Verification items for the finished model (mm, model axes). Coordinates: 2 decimals unless noted, no trailing zeros. Order: outer loops, then holes, each group sorted by start corner. A loop starts at its lowest first (then second) coordinate and runs counter-clockwise, first axis right, second up. Notation, with made-up numbers: M 27.5,36 L 69.5,36 A17 ccw 69.5,64 Z; hole C -17.75,-38.75 d10. An arc over 180 degrees is marked long. Return JSON: item names as keys, results as strings.
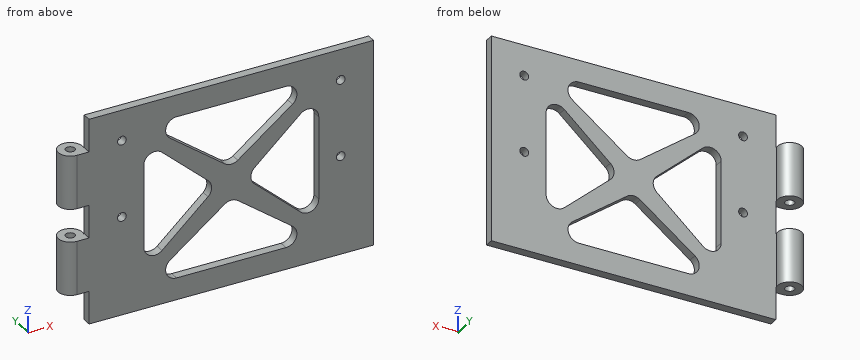
```python
from build123d import *

# Parameters (mm, degrees)
SKETCH_1_W           = 130
SKETCH_1_H           = 94
EXTRUDE_1_DEPTH      = 4
EXTRUDE_2_DEPTH      = 32
EXTRUDE_2_DEPTH_BACK = 32
SKETCH_4_R           = 2.1
CUT_EXTRUDE_1_DEPTH  = 122.379569945
SKETCH_10_W          = 11
SKETCH_10_H          = 15
CUT_EXTRUDE_2_DEPTH  = 24
CUT_EXTRUDE_3_DEPTH  = 10
SKETCH_12_R          = 2
CUT_EXTRUDE_4_DEPTH  = 10


with BuildPart() as part:
    # Эскиз1 → Бобышка-Вытянуть1 (new body)
    with BuildSketch(Plane(origin=(0, 0, 0), x_dir=(1, 0, 0), z_dir=(0, 1, 0))):
        Rectangle(SKETCH_1_W, SKETCH_1_H)
    extrude(amount=EXTRUDE_1_DEPTH)

    # Эскиз2 → Бобышка-Вытянуть2 (add, two sides: drawn at the far end of the back side and taken through both)
    with BuildSketch(Plane.XY.offset(-EXTRUDE_2_DEPTH_BACK)):
        with BuildLine():
            Line((-65, 4), (-65.208497378, 4))
            ThreePointArc((-65.208497378, 4), (-73.81662479, 9.887482194), (-70.5, 0))
            Line((-70.5, 0), (-65, 0))
            Line((-65, 0), (-65, 4))
        make_face()
    extrude(amount=EXTRUDE_2_DEPTH + EXTRUDE_2_DEPTH_BACK)

    # Эскиз4 → Вырез-Вытянуть1 (cut, through all)
    with BuildSketch(Plane.XY.offset(47)):
        with Locations((-70.5, 5.5)):
            Circle(SKETCH_4_R)
    extrude(amount=-CUT_EXTRUDE_1_DEPTH, mode=Mode.SUBTRACT)

    # Эскиз10 → Вырез-Вытянуть2 (cut)
    with BuildSketch(Plane(origin=(0, 0, 0), x_dir=(1, 0, 0), z_dir=(0, 1, 0))):
        with Locations((-70.5, 0)):
            Rectangle(SKETCH_10_W, SKETCH_10_H)
    extrude(amount=CUT_EXTRUDE_2_DEPTH, mode=Mode.SUBTRACT)

    # Эскиз11 → Вырез-Вытянуть3 (cut)
    with BuildSketch(Plane(origin=(0, 4, 0), x_dir=(1, 0, 0), z_dir=(0, 1, 0))):
        with BuildLine():
            Line((-25, 37), (25, 37))
            ThreePointArc((25, 37), (29.74341649, 33.58113883), (28, 28))
            Line((28, 28), (3, 9.25))
            ThreePointArc((3, 9.25), (0, 8.25), (-3, 9.25))
            Line((-3, 9.25), (-28, 28))
            ThreePointArc((-28, 28), (-29.74341649, 33.58113883), (-25, 37))
        make_face()
        with BuildLine():
            Line((-3, -9.25), (-28, -28))
            ThreePointArc((-28, -28), (-29.74341649, -33.58113883), (-25, -37))
            Line((-25, -37), (25, -37))
            ThreePointArc((25, -37), (29.74341649, -33.58113883), (28, -28))
            Line((28, -28), (3, -9.25))
            ThreePointArc((3, -9.25), (0, -8.25), (-3, -9.25))
        make_face()
        with BuildLine():
            Line((-10.625647004, 3.726779962), (-31.666666667, 22.546440075))
            ThreePointArc((-31.666666667, 22.546440075), (-37.041241452, 23.384014758), (-40, 18.819660113))
            Line((-40, 18.819660113), (-40, -18.819660113))
            ThreePointArc((-40, -18.819660113), (-37.041241452, -23.384014758), (-31.666666667, -22.546440075))
            Line((-31.666666667, -22.546440075), (-10.625647004, -3.726779962))
            ThreePointArc((-10.625647004, -3.726779962), (-8.958980338, 0), (-10.625647004, 3.726779962))
        make_face()
        with BuildLine():
            Line((10.625647004, 3.726779962), (31.666666667, 22.546440075))
            ThreePointArc((31.666666667, 22.546440075), (37.041241452, 23.384014758), (40, 18.819660113))
            Line((40, 18.819660113), (40, -18.819660113))
            ThreePointArc((40, -18.819660113), (37.041241452, -23.384014758), (31.666666667, -22.546440075))
            Line((31.666666667, -22.546440075), (10.625647004, -3.726779962))
            ThreePointArc((10.625647004, -3.726779962), (8.958980338, 0), (10.625647004, 3.726779962))
        make_face()
    extrude(amount=-CUT_EXTRUDE_3_DEPTH, mode=Mode.SUBTRACT)

    # Эскиз12 → Вырез-Вытянуть4 (cut)
    with BuildSketch(Plane(origin=(0, 4, 0), x_dir=(1, 0, 0), z_dir=(0, 1, 0))):
        with Locations(Location((-50, 2, 0), (0, 0, 270))):
            Circle(SKETCH_12_R)
        with Locations(Location((50, 2, 0), (0, 0, 270))):
            Circle(SKETCH_12_R)
        with Locations(Location((50, -33, 0), (0, 0, 270))):
            Circle(SKETCH_12_R)
        with Locations(Location((-50, -33, 0), (0, 0, 270))):
            Circle(SKETCH_12_R)
    extrude(amount=-CUT_EXTRUDE_4_DEPTH, mode=Mode.SUBTRACT)


solid = part.part
```
Q1. Cross-section at B-B, the plane y = 5.5. Record the boundary of the cut face in (x, z).
Values:
{"outline": "M -76,-32 L -72.6,-32 L -72.6,-7.5 L -76,-7.5 Z; M -76,7.5 L -72.6,7.5 L -72.6,32 L -76,32 Z; M -68.4,-32 L -65,-32 L -65,-7.5 L -68.4,-7.5 Z; M -68.4,7.5 L -65,7.5 L -65,32 L -68.4,32 Z"}
Q2. Cross-section at C-C, the plane z = -34. Record the boundary of the cut face in (x, y).
Values:
{"outline": "M -65,0 L -29.58,0 L -29.58,4 L -65,4 Z; M 29.58,0 L 65,0 L 65,4 L 29.58,4 Z"}
Q3. Material ranges on line 1 along Z through (x, y) = (-15.5, 0.5) (3 decimals); line 2 along X through (y, z) = (1.45, 33); line 3 along X through (y, z) = (2.9, -2), recorded low to high.
Values:
{"line 1": "-47 to -37, -18.625 to -8.087, 8.087 to 18.625, 37 to 47", "line 2": "-65 to -52, -48 to -29.9, 29.9 to 48, 52 to 65", "line 3": "-65 to -52, -48 to -40, -9.38 to 9.38, 40 to 48, 52 to 65"}
Q4. Go/stop test with flat-tipped pins: pin 1 (6.5 mm diameter, centred on x = -70.5, y = 5.5, fed in from +Z); pin 2 (2 mm diameter, centred on y = 2, z = -2, fed in from -X); pin 3 (5 mm diameter, centred on x = -50, z = -2, fed in from +Y). Record where each tip stops, or that it passes through.
Values:
{"pin 1": "z = 32", "pin 2": "x = -65", "pin 3": "y = 4"}
Q5. Cross-section at A-A, the plane x = -50. Record the boundary of the cut face in (y, z), and give its area (3 significant figures).
Values:
{"outline": "M 0,-47 L 4,-47 L 4,-4 L 0,-4 Z; M 0,0 L 4,0 L 4,31 L 0,31 Z; M 0,35 L 4,35 L 4,47 L 0,47 Z", "area": "344 mm^2"}
Q6. Cross-section at D-D, the plane x = 15.5. Record the boundary of the cut face in (y, z) (3 decimals), and give its area (3 significant figures).
Values:
{"outline": "M 0,-47 L 4,-47 L 4,-37 L 0,-37 Z; M 0,-18.625 L 4,-18.625 L 4,-8.087 L 0,-8.087 Z; M 0,8.087 L 4,8.087 L 4,18.625 L 0,18.625 Z; M 0,37 L 4,37 L 4,47 L 0,47 Z", "area": "164 mm^2"}
